Design review of the part shown in the three views and the two pictorial views. Dimensions are in mm from the part's minimum x, y and z. A direction names the side the tool comes from. Coordinates: 2 decimals unless noted, no trailing zeros. Loops run counter-clockwise (first coordinate to the right, second up) from the corner with the lowest first, then second, coordinate; pieces in that order, holes last. Notation, with made-up numbers: (18.25, -37) - (57.25, -37) arc R27 ccw to (57.25, -20) - close; hole circle Ø7 at (82, 77). An arc over 180 degrees is marked (long way). One line per question, with ' | ' between items.
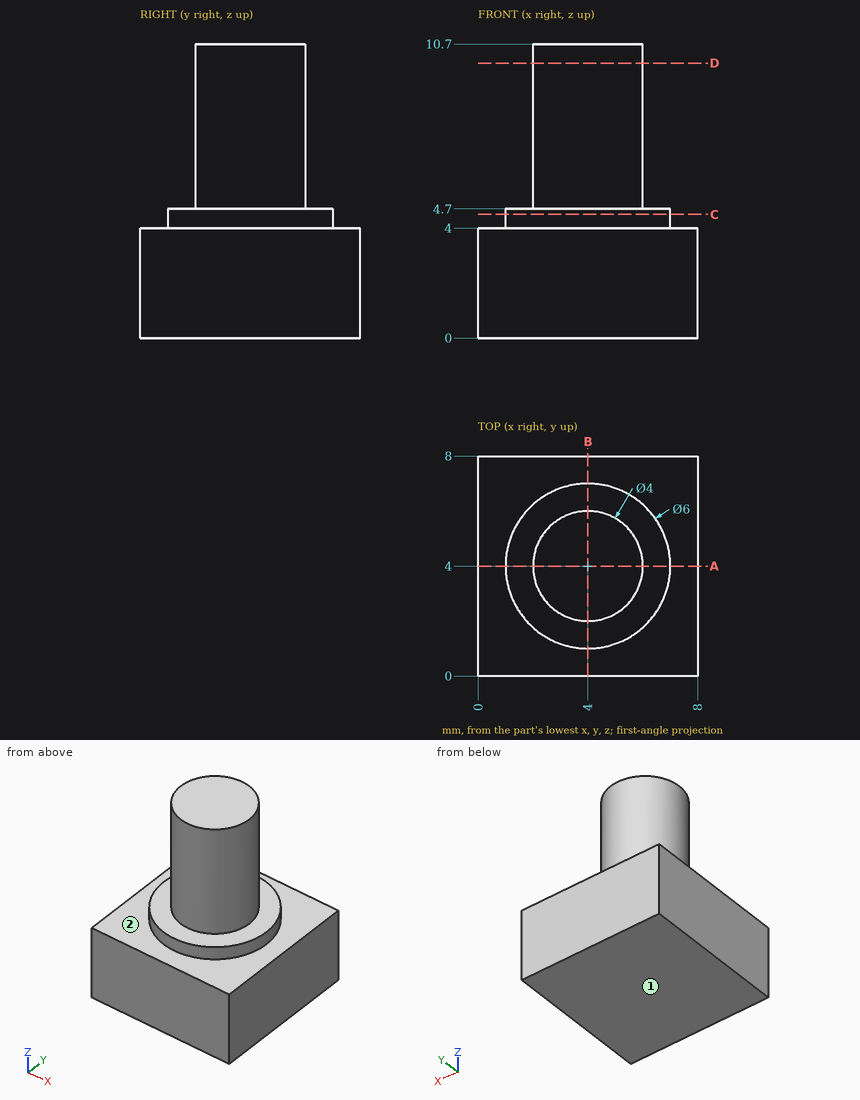
Q1. For pin 1 (1 mm diameter, centred on y = 2, z = 9, fed in from -X), flat-tipped, find the tip position at first contact; note if it passes through.
Returned:
pin 1: stops at x = 2.68
Q2. Take a section at C-C (z = 4.5). Give the boundary of the cut face in (x, y), plus the area to 3 significant figures.
Returned:
outline: circle Ø6 at (4, 4) | area: 28.3 mm²
Q3. Tool access review of the marked faces 1 and 2: name each direction out of +Z, -Z, +X, -X, +Y, -Y from which nothing blocks a thin tool from reaching the whole face with its end or side.
Returned:
face 1: -Z, +X, -X, +Y, -Y | face 2: +Z
Q4. To check wall thickness, follow line 1 along Y through (x, z) = (4, 9.5); line 2 along Z through (x, y) = (5.75, 6.5); line 3 along Z through (x, y) = (4, 1.25). State the ranges of each line that lie inside material, in increasing order.
Returned:
line 1: y = 2 to 6 | line 2: z = 0 to 4 | line 3: z = 0 to 4.7
Q5. Take a section at D-D (z = 10). Give the boundary of the cut face in (x, y).
Returned:
outline: circle Ø4 at (4, 4)
Q6. Take a section at A-A (y = 4). Give the boundary of the cut face in (x, z).
Returned:
outline: (0, 0) - (8, 0) - (8, 4) - (7, 4) - (7, 4.7) - (6, 4.7) - (6, 10.7) - (2, 10.7) - (2, 4.7) - (1, 4.7) - (1, 4) - (0, 4) - close
